from build123d import *

# Parameters (mm, degrees)
BOSS_EXTRUDE1_DEPTH = 5
SKETCH3_OUTSIDE_W   = 14.556
SKETCH3_OUTSIDE_H   = 8.356
SKETCH3_OUTSIDE_W_2 = 0.5
SKETCH3_OUTSIDE_H_2 = 0.3
SKETCH3_OUTSIDE_W_3 = 0.3
SKETCH3_OUTSIDE_H_3 = 3.8
CUT_EXTRUDE1_DEPTH  = 8.321885003
SKETCH4_W           = 0.5
SKETCH4_H           = 0.3
BOSS_EXTRUDE2_DEPTH = 2.9
SKETCH5_W           = 1.45
SKETCH5_H           = 0.3
SKETCH5_W_2         = 4.5
CUT_EXTRUDE2_DEPTH  = 1
SKETCH6_W           = 9.4
SKETCH6_H           = 3.2
SKETCH6_W_2         = 0.5
SKETCH6_H_2         = 0.3
CUT_EXTRUDE3_DEPTH  = 0.3
SKETCH7_W           = 9.4
SKETCH7_H           = 3.2
BOSS_EXTRUDE3_DEPTH = 0.7
SKETCH8_W           = 1
SKETCH8_H           = 1
BOSS_EXTRUDE4_DEPTH = 0.3
FILLET2_R           = 0.3
SKETCH9_W           = 4
SKETCH9_H           = 2.2
CUT_EXTRUDE4_DEPTH  = 0.3
SKETCH10_W          = 2
SKETCH10_H          = 2
BOSS_EXTRUDE5_DEPTH = 5.3
CUT_EXTRUDE5_DEPTH  = 12.285831826
SKETCH12_R          = 0.125
CUT_EXTRUDE6_DEPTH  = 0.1
SKETCH13_W          = 0.3
SKETCH13_H          = 0.3
CUT_EXTRUDE7_DEPTH  = 1.5


with BuildPart() as part:
    # Sketch2 → Boss-Extrude1 (new, symmetric)
    with BuildSketch(Plane(origin=(0, 0, 0), x_dir=(0, 0, -1), z_dir=(1, 0, 0))):
        with BuildLine():
            Line((-1.6, 5), (1.6, 5))
            ThreePointArc((1.6, 5), (1.812132034, 4.912132034), (1.9, 4.7))
            Line((1.9, 4.7), (1.9, 0))
            Line((1.9, 0), (1.487845372, 0))
            ThreePointArc((1.487845372, 0), (0.932721359, 0.496952053), (0.5, -0.109575967))
            Line((0.5, -0.109575967), (0.7, -1))
            Line((0.7, -1), (0.266442453, -1.837871024))
            ThreePointArc((0.266442453, -1.837871024), (0, -2), (-0.266442453, -1.837871024))
            Line((-0.266442453, -1.837871024), (-0.7, -1))
            Line((-0.7, -1), (-0.5, -0.109575967))
            ThreePointArc((-0.5, -0.109575967), (-0.932721359, 0.496952053), (-1.487845372, 0))
            Line((-1.487845372, 0), (-1.9, 0))
            Line((-1.9, 0), (-1.9, 4.7))
            ThreePointArc((-1.9, 4.7), (-1.812132034, 4.912132034), (-1.6, 5))
        make_face()
    extrude(amount=BOSS_EXTRUDE1_DEPTH, both=True)

    # Sketch3 outside → Cut-Extrude1 (cut, through all)
    with BuildSketch(Plane.XZ):
        Rectangle(SKETCH3_OUTSIDE_W, SKETCH3_OUTSIDE_H)
        with Locations((-2, 0)):
            Rectangle(SKETCH3_OUTSIDE_W_2, SKETCH3_OUTSIDE_H_2, mode=Mode.SUBTRACT)
        Rectangle(SKETCH3_OUTSIDE_W_2, SKETCH3_OUTSIDE_H_2, mode=Mode.SUBTRACT)
        with Locations((2, 0)):
            Rectangle(SKETCH3_OUTSIDE_W_2, SKETCH3_OUTSIDE_H_2, mode=Mode.SUBTRACT)
        with Locations((-4.85, 0)):
            Rectangle(SKETCH3_OUTSIDE_W_3, SKETCH3_OUTSIDE_H_3, mode=Mode.SUBTRACT)
        with Locations((4.85, 0)):
            Rectangle(SKETCH3_OUTSIDE_W_3, SKETCH3_OUTSIDE_H_3, mode=Mode.SUBTRACT)
    extrude(amount=CUT_EXTRUDE1_DEPTH, mode=Mode.SUBTRACT)

    # Sketch4 → Boss-Extrude2 (add)
    with BuildSketch(Plane.XZ):
        with Locations((-2, 0)):
            Rectangle(SKETCH4_W, SKETCH4_H)
        Rectangle(SKETCH4_W, SKETCH4_H)
        with Locations((2, 0)):
            Rectangle(SKETCH4_W, SKETCH4_H)
    extrude(amount=BOSS_EXTRUDE2_DEPTH)

    # Sketch5 → Cut-Extrude2 (cut)
    with BuildSketch(Plane.XZ):
        with Locations((-3.975, 1.75)):
            Rectangle(SKETCH5_W, SKETCH5_H)
        with Locations((0, 1.75)):
            Rectangle(SKETCH5_W_2, SKETCH5_H)
        with Locations((3.975, 1.75)):
            Rectangle(SKETCH5_W, SKETCH5_H)
        with Locations((3.975, -1.75)):
            Rectangle(SKETCH5_W, SKETCH5_H)
        with Locations((0, -1.75)):
            Rectangle(SKETCH5_W_2, SKETCH5_H)
        with Locations((-3.975, -1.75)):
            Rectangle(SKETCH5_W, SKETCH5_H)
    extrude(amount=-CUT_EXTRUDE2_DEPTH, mode=Mode.SUBTRACT)

    # Sketch6 → Cut-Extrude3 (cut)
    with BuildSketch(Plane.XZ):
        Rectangle(SKETCH6_W, SKETCH6_H)
        with Locations((-2, 0)):
            Rectangle(SKETCH6_W_2, SKETCH6_H_2, mode=Mode.SUBTRACT)
        Rectangle(SKETCH6_W_2, SKETCH6_H_2, mode=Mode.SUBTRACT)
        with Locations((2, 0)):
            Rectangle(SKETCH6_W_2, SKETCH6_H_2, mode=Mode.SUBTRACT)
    extrude(amount=-CUT_EXTRUDE3_DEPTH, mode=Mode.SUBTRACT)

    # Sketch7 → Boss-Extrude3 (add)
    with BuildSketch(Plane.XZ.offset(-0.3)):
        Rectangle(SKETCH7_W, SKETCH7_H)
    extrude(amount=-BOSS_EXTRUDE3_DEPTH)

    # Sketch8 → Boss-Extrude4 (add)
    with BuildSketch(Plane.XZ):
        with Locations((-2.75, 1.4)):
            Rectangle(SKETCH8_W, SKETCH8_H)
        with Locations((2.75, 1.4)):
            Rectangle(SKETCH8_W, SKETCH8_H)
        with Locations((2.75, -1.4)):
            Rectangle(SKETCH8_W, SKETCH8_H)
        with Locations((-2.75, -1.4)):
            Rectangle(SKETCH8_W, SKETCH8_H)
    extrude(amount=-BOSS_EXTRUDE4_DEPTH)

    # Fillet2
    # the kernel refuses this fillet: 0.3 mm, written as the material it takes off along each edge
    with BuildSketch(Plane(origin=(-5, 5, 2.35), x_dir=(1, 0, 0), z_dir=(0, 0, -1)), Plane(origin=(5, 5, 2.35), x_dir=(0, -1, 0), z_dir=(0, 0, -1))) as fillet2_piece_1:
        with BuildLine():
            CenterArc((FILLET2_R, FILLET2_R), FILLET2_R, 180, 90)
            Line((0, FILLET2_R), (0, 0))
            Line((0, 0), (FILLET2_R, 0))
        make_face()
    extrude(amount=4.7, mode=Mode.SUBTRACT)
    with BuildSketch(Plane(origin=(1.5, 0, 1.9), x_dir=(0, 0, -1), z_dir=(1, 0, 0)), Plane(origin=(-4, 0, 1.9), x_dir=(0, 0, -1), z_dir=(1, 0, 0))) as fillet2_piece_2:
        with BuildLine():
            CenterArc((FILLET2_R, FILLET2_R), FILLET2_R, 180, 90)
            Line((0, FILLET2_R), (0, 0))
            Line((0, 0), (FILLET2_R, 0))
        make_face()
    extrude(amount=2.5, mode=Mode.SUBTRACT)
    with BuildSketch(Plane(origin=(1.5, 0, -1.9), x_dir=(0, 0, 1), z_dir=(1, 0, 0)), Plane(origin=(-4, 0, -1.9), x_dir=(0, 0, 1), z_dir=(1, 0, 0))) as fillet2_piece_3:
        with BuildLine():
            CenterArc((FILLET2_R, -FILLET2_R), FILLET2_R, 90, 90)
            Line((0, -FILLET2_R), (0, 0))
            Line((0, 0), (FILLET2_R, 0))
        make_face()
    extrude(amount=2.5, mode=Mode.SUBTRACT)

    # Sketch9 → Cut-Extrude4 (cut)
    with BuildSketch(Plane.XY.offset(1.9)):
        with Locations((0, 3.5)):
            Rectangle(SKETCH9_W, SKETCH9_H)
    extrude(amount=-CUT_EXTRUDE4_DEPTH, mode=Mode.SUBTRACT)

    # Sketch10 → Boss-Extrude5 (add)
    with BuildSketch(Plane.XY.offset(1.6)):
        with Locations((1, 3.5)):
            Rectangle(SKETCH10_W, SKETCH10_H)
    extrude(amount=BOSS_EXTRUDE5_DEPTH)

    # Sketch11 → Cut-Extrude5 (cut, through all)
    with BuildSketch(Plane(origin=(0, 4.5, 0), x_dir=(1, 0, 0), z_dir=(0, 1, 0))):
        Polygon((0, -6.6), (0.25, -6.9), (0.5, -6.6), (0.75, -6.9), (1, -6.6), (1.25, -6.9), (1.5, -6.6), (1.75, -6.9), (2, -6.6), (2.5, -6.6), (2.5, -7.4), (-0.5, -7.4), (-0.5, -6.6), align=None)
    extrude(amount=-CUT_EXTRUDE5_DEPTH, mode=Mode.SUBTRACT)

    # Sketch12 → Cut-Extrude6 (cut)
    with BuildSketch(Plane.XZ.offset(2.9)):
        with Locations(Location((-2, 0, 0), (0, 0, 270))):
            Circle(SKETCH12_R)
        with Locations(Location((2, 0, 0), (0, 0, 270))):
            Circle(SKETCH12_R)
    extrude(amount=-CUT_EXTRUDE6_DEPTH, mode=Mode.SUBTRACT)

    # Sketch13 → Cut-Extrude7 (cut)
    with BuildSketch(Plane(origin=(0, 5, 0), x_dir=(1, 0, 0), z_dir=(0, 1, 0))):
        with Locations((-4.85, -1.75)):
            Rectangle(SKETCH13_W, SKETCH13_H)
        with Locations((-4.85, 1.75)):
            Rectangle(SKETCH13_W, SKETCH13_H)
        with Locations((4.85, 1.75)):
            Rectangle(SKETCH13_W, SKETCH13_H)
        with Locations((4.85, -1.75)):
            Rectangle(SKETCH13_W, SKETCH13_H)
    extrude(amount=-CUT_EXTRUDE7_DEPTH, mode=Mode.SUBTRACT)


solid = part.part
The listing builds one solid part. Answer for the finished solid, in the listing's coordinates (mm). A direction names the side the tool comes from. Coordinates: 2 decimals unless noted, no trailing zeros. Loops run counter-clockwise (first coordinate to the right, second up) from the corner with the lowest first, then second, coordinate; pieces in that order, holes last.
1) Find section C-C on x = 4. Write down the section's boundary in (y, z), then the cut area to 3 significant figures.
2) Determine the mould class of faces 1 (the face through (0, 5, 0)), 2 (the face through (5, 2, 0)), 3 (the face through (-1, 4, 1.6)) for opening direction X: pulls with the +X half, pulls with the -X half, needs draft (parallel to the pull), parting line crosses it, or undercut.
3) Find the intervals of material crossed by L1, parallel to Y at x = 3.75, z = -0.25; L2, parallel to Z at x = 3, y = 0.75; L3, parallel to Y at x = 0.75, z = 2.75, in increasing order.
4) Flat-ended cylindrical pins translate along their axes: pin 1 Ø2 at (x, z) = (0, 2.5) entering from -Y; pin 2 Ø0.6 at (x, z) = (2.5, 1) entering from -Y; pin 3 Ø0.6 at (x, z) = (1, 3) entering from +Y. Find the tip coordinate at first contact, or state that the pin passes through.
5) Find section D-D on y = 2.75. Write down the section's boundary in (x, z), then the cut area to 3 significant figures.
6) A tool of negligible diameter and unlimited length cuts with its end or side. For faces 4 (the face through (0, 3, -1.9)), 5 (the face through (-4.7, -1, 0)), 6 (the face through (-0.1, 0.3, 0.4)), from which of +Z, -Z, +X, -X, +Y, -Y can it reach the whole face along a straight path? Write none if from no direction.
7) Find section A-A on y = -0.5. Write down the section's boundary in (x, z), then the cut area to 3 significant figures.
Values:
1. outline: (0.3, -1.6) - (1, -1.6) - (1, -1.9) - (4.7, -1.9) arc R0.3 ccw to (5, -1.6) - (5, 1.6) arc R0.3 ccw to (4.7, 1.9) - (1, 1.9) - (1, 1.6) - (0.3, 1.6) - close
1. area: 17.4 mm2
2. face 1: needs draft
2. face 2: pulls with the +X half
2. face 3: undercut
3. L1: y = 0.3 to 5
3. L2: z = -1.9 to 1.9
3. L3: y = 2.5 to 4.5
4. pin 1: stops at y = 0.3
4. pin 2: stops at y = 0
4. pin 3: stops at y = 4.5
5. outline: (-5, -1.9) - (5, -1.9) - (5, 1.9) - (2, 1.9) - (2, 6.6) - (1.75, 6.9) - (1.5, 6.6) - (1.25, 6.9) - (1, 6.6) - (0.75, 6.9) - (0.5, 6.6) - (0.25, 6.9) - (0, 6.6) - (0, 1.6) - (-2, 1.6) - (-2, 1.9) - (-5, 1.9) - close
5. area: 47.1 mm2
6. face 4: -Z, +X, -X, +Y, -Y
6. face 5: +Z, -Z, -Y
6. face 6: -Y
7. outline: (-5, -0.59) - (-4.7, -0.59) - (-4.7, 0.59) - (-5, 0.59) - close; (-2.25, -0.15) - (-1.75, -0.15) - (-1.75, 0.15) - (-2.25, 0.15) - close; (-0.25, -0.15) - (0.25, -0.15) - (0.25, 0.15) - (-0.25, 0.15) - close; (1.75, -0.15) - (2.25, -0.15) - (2.25, 0.15) - (1.75, 0.15) - close; (4.7, -0.59) - (5, -0.59) - (5, 0.59) - (4.7, 0.59) - close
7. area: 1.16 mm2
